from build123d import *

# Parameters (mm, degrees)
F0_W     = 152.7
F0_H     = 74.7
F1_DEPTH = 7.25
F2_R     = 8
F3_SIZE  = 1
F4_R     = 3.5


with BuildPart() as f1:
    # F0 (on Top) → F1 (new body)
    with BuildSketch(Plane.XY):
        Rectangle(F0_W, F0_H)
    extrude(amount=F1_DEPTH)

    # F2
    f2_edges = [f1.edges().sort_by_distance(p)[0] for p in [
        (-76.35, -37.35, 3.625),
        (76.35, -37.35, 3.625),
        (76.35, 37.35, 3.625),
        (-76.35, 37.35, 3.625),
    ]]
    fillet(f2_edges, radius=F2_R)

    # F3
    f3_edges = [f1.edges().sort_by_distance(p)[0] for p in [
        (0, -37.35, 0),
        (74.006854, -35.006854, 0),
        (76.35, 0, 0),
        (74.006854, 35.006854, 0),
        (-74.006854, -35.006854, 0),
        (-76.35, 0, 0),
        (-74.006854, 35.006854, 0),
        (0, 37.35, 0),
    ]]
    chamfer(f3_edges, length=F3_SIZE)

    # F4
    f4_edges = [f1.edges().sort_by_distance(p)[0] for p in [
        (0, -37.35, 7.25),
    ]]
    fillet(f4_edges, radius=F4_R)


solid = f1.part
The listing builds one solid part. Answer for the finished solid, in the listing's coordinates (mm). Coordinates: 2 decimals unless noted, no trailing zeros. Order: outer loops, then holes, each group sorted by start corner. A loop starts at its lowest first (then second) coordinate and runs counter-clockwise, first axis right, second up.
Q1. A cutting plane is placed at A-A, the plane z = 6. Write down the section's boundary in (x, y).
Q2. Given P1, Ø1, axis at x = -21, z = 4.5, coming from the -Y side; P2, Ø1.5, axis at y = -3, z = 6.5, coming from the -X side; P3, Ø2, axis at y = 7, z = 5.5, coming from the -X side, each flat-ended and moving along its own axis, determine where each tip first touches the part or whether it passes through.
Q3. Consider line 1 (X direction, y = 29, z = 4); line 2 (Y direction, x = 39, z = 0.5); line 3 (X direction, y = -32, z = 4). Determine where each line is inside the solid, lowest interval first.
Answers follow:
1. outline: (-75.53, -29.35) arc R7.18 ccw to (-68.35, -36.53) - (68.35, -36.53) arc R7.18 ccw to (75.53, -29.35) - (75.53, 29.35) arc R7.18 ccw to (68.35, 36.53) - (-68.35, 36.53) arc R7.18 ccw to (-75.53, 29.35) - close
2. P1: stops at y = -37.34
2. P2: stops at x = -75.72
2. P3: stops at x = -76.27
3. line 1: x = -76.34 to 76.34
3. line 2: y = -36.85 to 36.85
3. line 3: x = -75.89 to 75.89
